from build123d import *

# Parameters (mm, degrees)
F1_DEPTH = 25.4
F3_DEPTH = 76.2
F4_R     = 4.699
F5_DEPTH = 25.4


with BuildPart() as f1:
    # F0 (on Front) → F1 (new body)
    with BuildSketch(Plane.XZ):
        Polygon((-36.353452, 38.035411), (-60.178652, 38.035411), (-60.178652, -12.764589), (16.046748, -12.764589), (16.046748, 38.035411), (-7.778452, 38.035411), (-7.778452, 9.460411), (-36.353452, 9.460411), align=None)
    extrude(amount=F1_DEPTH)

    # F2 (on face) → F3 (join)
    with BuildSketch(Plane(origin=(-60.178652, 0, 0), x_dir=(0, -1, 0), z_dir=(-1, 0, 0))):
        Polygon((50.8, -12.764589), (0, -12.764589), (-44.45, -12.764589), (-44.45, -31.814589), (50.8, -31.814589), align=None)
    extrude(amount=-F3_DEPTH)

    # F4 (on face) → F5 (cut)
    with BuildSketch(Plane.XY.offset(-12.764589)):
        with Locations((3.321348, 31.75)):
            Circle(F4_R)
        with Locations((-47.478652, 31.75)):
            Circle(F4_R)
        with Locations((-47.478652, -38.1)):
            Circle(F4_R)
        with Locations((3.321348, -38.1)):
            Circle(F4_R)
    extrude(amount=-F5_DEPTH, mode=Mode.SUBTRACT)


solid = f1.part
Work out the finished part from the listing and answer in its coordinate system (mm). A direction names the side the tool comes from. Round coordinates to 2 decimals unless told otherwise and drop trailing zeros. Loops run counter-clockwise (first coordinate to the right, second up) from the corner with the lowest first, then second, coordinate; pieces in that order, holes last. Notation, with made-up numbers: (55.25, 75) -> (90.25, 75) arc R25 cw to (90.25, 113) -> close; hole circle Ø5 at (-24.5, -2.75). An arc over 180 degrees is marked (long way). Use one line per item in the form item = value.
(1) Find section B-B on y = 31.75. Give the vertices of the cut face in (x, z), then the cut area to 3 significant figures.
Answer list:
outline = (-60.18, -31.81) -> (-52.18, -31.81) -> (-52.18, -12.76) -> (-60.18, -12.76) -> close; (-42.78, -31.81) -> (-1.38, -31.81) -> (-1.38, -12.76) -> (-42.78, -12.76) -> close; (8.02, -31.81) -> (16.02, -31.81) -> (16.02, -12.76) -> (8.02, -12.76) -> close
area = 1,090 mm2
(2) Straight lines are drawn through the part: line 1 (X direction, y = -38, z = -25); line 2 (X direction, y = 31, z = -19); line 3 (X direction, y = 20, z = -27). For each, find the intervals that lie inside material, in ascending order.
Answer list:
line_1 = -60.18 to -52.18, -42.78 to -1.38, 8.02 to 16.02
line_2 = -60.18 to -52.12, -42.84 to -1.32, 7.96 to 16.02
line_3 = -60.18 to 16.02
(3) Find section D-D on x = -3.5. Give the vertices of the cut face in (y, z).
Answer list:
outline = (-50.8, -31.81) -> (44.45, -31.81) -> (44.45, -12.76) -> (0, -12.76) -> (0, 38.04) -> (-25.4, 38.04) -> (-25.4, -12.76) -> (-50.8, -12.76) -> close
(4) Find section A-A on z = 32.5. Give the vertices of the cut face in (x, y), then the cut area to 3 significant figures.
Answer list:
outline = (-60.18, -25.4) -> (-36.35, -25.4) -> (-36.35, 0) -> (-60.18, 0) -> close; (-7.78, -25.4) -> (16.05, -25.4) -> (16.05, 0) -> (-7.78, 0) -> close
area = 1,210 mm2
(5) Find section C-C on z = -15.5. Give the vertices of the cut face in (x, y).
Answer list:
outline = (-60.18, -50.8) -> (16.02, -50.8) -> (16.02, 44.45) -> (-60.18, 44.45) -> close; hole circle Ø9.4 at (-47.48, -38.1); hole circle Ø9.4 at (-47.48, 31.75); hole circle Ø9.4 at (3.32, -38.1); hole circle Ø9.4 at (3.32, 31.75)
(6) For a pull along X with two mould halves and no side action, classify faces 4 (the flat face through (-36.353, -13, 24)), 5 (the cylindrical face through (-42.997, 33.161, -22.156)), 6 (the flat face through (-23, -38, -12.765)), 7 (the flat face through (16.021, -3, -22)) as released by +X, released by -X, zero draft, split by the parting line, or undercut.
Answer list:
face_4 = undercut
face_5 = undercut
face_6 = zero draft
face_7 = released by +X
(7) Flat-ended cylindrical pins translate along their axes: P1, Ø7.5, axis at x = 3.32, y = 31.75, coming from the -Z side; P2, Ø15, axis at y = -21, z = -27, coming from the +X side; P3, Ø15, axis at x = -16.5, z = 0.5, coming from the -Y side; P4, Ø4, axis at x = -34.5, y = 18, coming from the +Z side. Find the tip coordinate at first contact, or state that the pin passes through.
Answer list:
P1 = through
P2 = 16.02
P3 = -25.4
P4 = -12.76
(8) A tool of negligible diameter and unlimited length cuts with its end or side. For faces 1 (the flat face through (-23, -25.4, 7)), 2 (the flat face through (-22, -13, 9.46)), 3 (the flat face through (-23, 0, 7)), from which of +Z, -Z, +X, -X, +Y, -Y can it reach the whole face along a straight path? Write none if from no direction.
Answer list:
face_1 = +Z, +X, -X, -Y
face_2 = +Z, +Y, -Y
face_3 = +Z, +X, -X, +Y
